The model under review builds one solid part; all positions refer to its coordinate system, in mm. Face numbers are marked on the shaded views. A direction names the side the tool comes from. Round coordinates to 2 decimals unless told otherwise and drop trailing zeros. Order: outer loops, then holes, each group sorted by start corner. A loop starts at its lowest first (then second) coordinate and runs counter-clockwise, first axis right, second up. Notation, with made-up numbers: M 68.5,73 L 111.5,73 A25 cw 111.5,112 Z; hole C -31.75,20 d3. An arc over 180 degrees is marked long. Answer as a JSON object with one key per item and string values. Group by question number.
1. Add section C-C on z = 10. State the section outline as (x, y) points.
2. Clearance check with flat-ended pins moving along their axes: P1, Ø3, axis at y = 34.5, z = 19.5, coming from the +X side; P2, Ø1.5, axis at x = 12.5, y = 38.5, coming from the -Z side; P3, Ø4, axis at x = 29, z = 7, coming from the +Y side. State where each tip first meets the part, or that it passes through.
3. Machinability: for the marked faces 1 and 2, which of the approach directions +Z, -Z, +X, -X, +Y, -Y give a long, thin tool a straight path to every point of the face, cutting with its end or side? Answer none if there is none.
4. To check wall thickness, follow probe 1 along Y at (x, z) = (35, 24.15); probe 2 along Z at (x, y) = (10, 23.5); probe 3 along X at (y, z) = (8.5, 6.75). State the ranges of each line that lie inside material, in increasing order. Write a range as [from, to].
5. Add section D-D on y = 24. State the section outline as (x, z) points.
6. Add section A-A on y = 35. State the section outline as (x, z) points.
```python
from build123d import *

# Parameters (mm, degrees)
SKETCH001_W  = 42
SKETCH001_H  = 42
PAD001_DEPTH = 26
SKETCH_W     = 45
SKETCH_H     = 45
PAD_DEPTH    = 26
SKETCH002_R  = 1
POCKET_DEPTH = 26.001


with BuildPart() as obj1:
    # Sketch001 → Pad001 (new body)
    with BuildSketch(Plane.XY):
        with Locations((21, 21)):
            Rectangle(SKETCH001_W, SKETCH001_H)
    extrude(amount=PAD001_DEPTH)


with BuildPart() as obj1_1:
    # Body001 placement: moved
    add(obj1.part.moved(Location((3, 3, -3))))


with BuildPart() as obj2:
    # Sketch → Pad (new body)
    with BuildSketch(Plane.XY):
        with Locations((22.5, 22.5)):
            Rectangle(SKETCH_W, SKETCH_H)
    extrude(amount=PAD_DEPTH)

    # Boolean: cut obj1
    add(obj1_1.part, mode=Mode.SUBTRACT)

    # Sketch002 (on Face6 of Boolean) → Pocket (cut, through all)
    with BuildSketch(Plane.XY.offset(26)):
        with Locations((35, 35)):
            Circle(SKETCH002_R)
    extrude(amount=-POCKET_DEPTH, mode=Mode.SUBTRACT)


solid = obj2.part
```
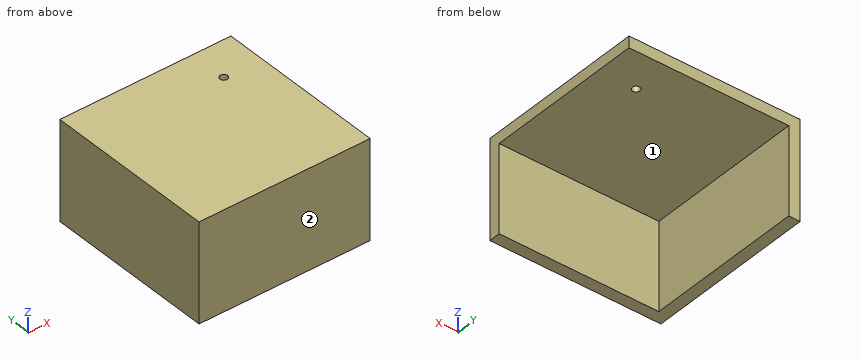
Recorded:
{
 "1": {"outline": "M 0,0 L 45,0 L 45,3 L 3,3 L 3,45 L 0,45 Z"},
 "2": {"P1": "stops at x = 3", "P2": "stops at z = 23", "P3": "stops at y = 3"},
 "3": {"face 1": "-Z, +X, +Y", "face 2": "+Z, -Z, +X, -X, -Y"},
 "4": {"probe 1": "y = [0, 34], [36, 45]", "probe 2": "z = [23, 26]", "probe 3": "x = [0, 3]"},
 "5": {"outline": "M 0,0 L 3,0 L 3,23 L 45,23 L 45,26 L 0,26 Z"},
 "6": {"outline": "M 0,0 L 3,0 L 3,23 L 34,23 L 34,26 L 0,26 Z; M 36,23 L 45,23 L 45,26 L 36,26 Z"}
}
